Geometry: final body of the model. Coordinates: model frame, mm. A direction names the side the tool comes from. Round coordinates to 2 decimals unless told otherwise and drop trailing zeros. Loops run counter-clockwise (first coordinate to the right, second up) from the corner with the lowest first, then second, coordinate; pieces in that order, holes last. Notation, with made-up numbers: M 56.5,8.5 L 93.5,8.5 A24 ccw 93.5,29.5 Z; hole C 24.5,88 d5. An arc over 180 degrees is marked long. Answer as a JSON object with one key per item and string values.
```python
from build123d import *

# Parameters (mm, degrees)
F0_R     = 9
F0_R_2   = 4
F1_DEPTH = 1
F2_R     = 4
F3_DEPTH = 0.25


with BuildPart() as f1:
    # F0 (on Top) → F1 (new body)
    with BuildSketch(Plane.XY):
        Circle(F0_R)
        Circle(F0_R_2, mode=Mode.SUBTRACT)
    extrude(amount=F1_DEPTH)

    # F2 (on face) → F3 (cut)
    with BuildSketch(Plane(origin=(0, 0, 0), x_dir=(1, 0, 0), z_dir=(0, 0, -1))):
        with BuildLine():
            ThreePointArc((4.875, 7.5653403757), (2.5408597579, 8.6338885614), (0, 9))
            ThreePointArc((0, 9), (-2.5408597579, 8.6338885614), (-4.875, 7.5653403757))
            Line((-4.875, 7.5653403757), (-4.875, -7.5653403757))
            ThreePointArc((-4.875, -7.5653403757), (-2.5408597579, -8.6338885614), (0, -9))
            ThreePointArc((0, -9), (2.5408597579, -8.6338885614), (4.875, -7.5653403757))
            Line((4.875, -7.5653403757), (4.875, 7.5653403757))
        make_face()
        Circle(F2_R, mode=Mode.SUBTRACT)
        Circle(F2_R)
    extrude(amount=-F3_DEPTH, mode=Mode.SUBTRACT)


solid = f1.part
```
1) Pull-direction query (Y, two-part tool) for faces 1 (the face through (-0.867, -3.905, 0.62)), 2 (the face through (4, -2, 1)), 3 (the face through (-8.99, 0.4, 0.49)); classes: +Y half, -Y half, draft (parallel to the pull), parting line (faces both ways), or undercut.
Geometry results:
{"face 1": "undercut", "face 2": "draft", "face 3": "parting line"}
2) Set-up query: faces 4 (the face through (1, -4.1, 0.25)), 5 (the face through (6, 0, 0)). Return all of +Z, -Z, +X, -X, +Y, -Y with unobstructed straight access to the full face (end or side cutting, diameter ignored); none if empty.
Geometry results:
{"face 4": "-Z, +Y, -Y", "face 5": "-Z, +X, -X, +Y, -Y"}
3) Cut plane D-D on y = 7.25. Return the cut outline in (x, z) (3 decimals).
Geometry results:
{"outline": "M -5.333,0 L -4.875,0 L -4.875,0.25 L 4.875,0.25 L 4.875,0 L 5.333,0 L 5.333,1 L -5.333,1 Z"}
4) Cut plane C-C on z = 0.8. Return the cut outline in (x, y).
Geometry results:
{"outline": "C 0,0 d18; hole C 0,0 d8"}
5) Cut plane A-A on y = 0. Return the cut outline in (x, z) (3 decimals).
Geometry results:
{"outline": "M -9,0 L -4.875,0 L -4.875,0.25 L -4,0.25 L -4,1 L -9,1 Z; M 4,0.25 L 4.875,0.25 L 4.875,0 L 9,0 L 9,1 L 4,1 Z"}
6) First-contact query: pin 1 (4 mm diameter, centred on x = -0.5, y = 6.5, fed in from -Z); pin 2 (3 mm diameter, centred on x = -4.5, y = 3.5, fed in from -Z). Flat tips, straight axial feed; report the tip coordinate or a pass-through.
Geometry results:
{"pin 1": "z = 0.25", "pin 2": "z = 0"}
7) Cut plane B-B on x = 0. Return the cut outline in (y, z).
Geometry results:
{"outline": "M -9,0.25 L -4,0.25 L -4,1 L -9,1 Z; M 4,0.25 L 9,0.25 L 9,1 L 4,1 Z"}
8) Line query: probe 1 along X at (y, z) = (0, 0.6); probe 2 along Z at (x, y) = (0.75, 5). Output: solid intervals per line, ascending.
Geometry results:
{"probe 1": "-9 to -4, 4 to 9", "probe 2": "0.25 to 1"}
